Geometry: final body of the model. Coordinates: model frame, mm. Face numbers are marked on the shaded views. A direction names the side the tool comes from. Round coordinates to 2 decimals unless told otherwise and drop trailing zeros. Loops run counter-clockwise (first coordinate to the right, second up) from the corner with the lowest first, then second, coordinate; pieces in that order, holes last. Notation, with made-up numbers: M 3.25,67 L 54.25,67 A25 ccw 54.25,97 Z; hole C 52,-35.5 d3. An arc over 180 degrees is marked long. Answer as a JSON object with one key per item and string values.
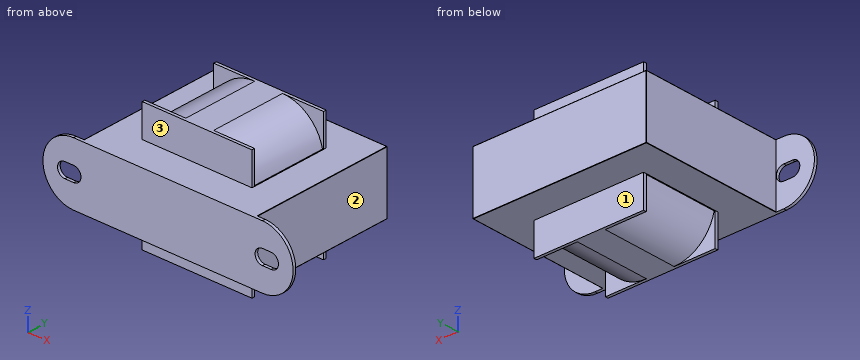
from build123d import *

# Parameters (mm, degrees)
SKETCH1_W           = 59.3
SKETCH1_H           = 48.97
BASE_EXTRUDE_DEPTH  = 10.5
BOSS_EXTRUDE1_DEPTH = 1
CUT_EXTRUDE1_DEPTH  = 10
BOSS_EXTRUDE2_DEPTH = 13
CUT_EXTRUDE2_DEPTH  = 13
SKETCH6_W           = 37.5
SKETCH6_H           = 43
BOSS_EXTRUDE3_DEPTH = 1
SKETCH7_W           = 37.5
SKETCH7_H           = 43
BOSS_EXTRUDE4_DEPTH = 1
FILLET1_R           = 0.1


with BuildPart() as part:
    # Sketch1 → Base-Extrude (new body, symmetric)
    with BuildSketch(Plane.XY):
        with Locations((32.25, 25.485)):
            Rectangle(SKETCH1_W, SKETCH1_H)
    extrude(amount=BASE_EXTRUDE_DEPTH, both=True)

    # Sketch2 → Boss-Extrude1 (add)
    with BuildSketch(Plane.XZ.offset(-1)):
        with BuildLine():
            Line((0, 10.5), (64.5, 10.5))
            ThreePointArc((64.5, 10.5), (75, 0), (64.5, -10.5))
            Line((64.5, -10.5), (0, -10.5))
            ThreePointArc((0, -10.5), (-10.5, 0), (0, 10.5))
        make_face()
    extrude(amount=BOSS_EXTRUDE1_DEPTH)

    # Sketch3 → Cut-Extrude1 (cut)
    with BuildSketch(Plane.XZ):
        with BuildLine():
            Line((64.5, 2.5), (67.5, 2.5))
            ThreePointArc((67.5, 2.5), (70, 0), (67.5, -2.5))
            Line((67.5, -2.5), (64.5, -2.5))
            ThreePointArc((64.5, -2.5), (62, 0), (64.5, 2.5))
        make_face()
        with BuildLine():
            Line((-3, 2.5), (0, 2.5))
            ThreePointArc((0, 2.5), (2.5, 0), (0, -2.5))
            Line((0, -2.5), (-3, -2.5))
            ThreePointArc((-3, -2.5), (-5.5, 0), (-3, 2.5))
        make_face()
    extrude(amount=-CUT_EXTRUDE1_DEPTH, mode=Mode.SUBTRACT)

    # Sketch4 → Boss-Extrude2 (add, symmetric)
    with BuildSketch(Plane(origin=(0, 24.97, 0), x_dir=(-1, 0, 0), z_dir=(0, 1, 0))):
        with BuildLine():
            Line((-37, 21.5), (-27.5, 21.5))
            ThreePointArc((-27.5, 21.5), (-17.600505063, 17.399494937), (-13.5, 7.5))
            Line((-13.5, 7.5), (-13.5, -7.5))
            ThreePointArc((-13.5, -7.5), (-17.600505063, -17.399494937), (-27.5, -21.5))
            Line((-27.5, -21.5), (-37, -21.5))
            ThreePointArc((-37, -21.5), (-46.899494937, -17.399494937), (-51, -7.5))
            Line((-51, -7.5), (-51, 7.5))
            ThreePointArc((-51, 7.5), (-46.899494937, 17.399494937), (-37, 21.5))
        make_face()
    extrude(amount=BOSS_EXTRUDE2_DEPTH, both=True)

    # Sketch5 → Cut-Extrude2 (cut, symmetric)
    with BuildSketch(Plane(origin=(0, 24.97, 0), x_dir=(-1, 0, 0), z_dir=(0, 1, 0))):
        with BuildLine():
            Line((-13.5, 10.5), (-13.825205669, 10.5))
            ThreePointArc((-13.825205669, 10.5), (-13.581538867, 9.008787487), (-13.5, 7.5))
            Line((-13.5, 7.5), (-13.5, 10.5))
        make_face()
        with BuildLine():
            Line((-51, 10.5), (-50.674794331, 10.5))
            ThreePointArc((-50.674794331, 10.5), (-50.918461133, 9.008787487), (-51, 7.5))
            Line((-51, 7.5), (-51, 10.5))
        make_face()
        with BuildLine():
            Line((-51, -10.5), (-50.674794331, -10.5))
            ThreePointArc((-50.674794331, -10.5), (-50.918461133, -9.008787487), (-51, -7.5))
            Line((-51, -7.5), (-51, -10.5))
        make_face()
        with BuildLine():
            Line((-13.5, -10.5), (-13.825205669, -10.5))
            ThreePointArc((-13.825205669, -10.5), (-13.581538867, -9.008787487), (-13.5, -7.5))
            Line((-13.5, -7.5), (-13.5, -10.5))
        make_face()
    extrude(amount=CUT_EXTRUDE2_DEPTH, both=True, mode=Mode.SUBTRACT)

    # Sketch6 → Boss-Extrude3 (add)
    with BuildSketch(Plane(origin=(0, 37.97, 0), x_dir=(-1, 0, 0), z_dir=(0, 1, 0))):
        with Locations((-32.25, 0)):
            Rectangle(SKETCH6_W, SKETCH6_H)
    extrude(amount=BOSS_EXTRUDE3_DEPTH)

    # Sketch7 → Boss-Extrude4 (add)
    with BuildSketch(Plane.XZ.offset(-11.97)):
        with Locations((32.25, 0)):
            Rectangle(SKETCH7_W, SKETCH7_H)
    extrude(amount=BOSS_EXTRUDE4_DEPTH)

    # Fillet1
    fillet1_edges = [part.edges().sort_by_distance(p)[0] for p in [
        (61.9, 25.485, 10.5),
        (32.25, 49.97, 10.5),
        (2.6, 25.485, 10.5),
        (32.25, 49.97, -10.5),
        (61.9, 25.485, -10.5),
        (2.6, 25.485, -10.5),
        (2.6, 49.97, 0),
        (61.9, 49.97, 0),
    ]]
    fillet(fillet1_edges, radius=FILLET1_R)


solid = part.part
1) Section query A-A (z = 0). Return the cut outline in (x, y).
Results:
{"outline": "M -10.5,0 L -5.5,0 L -5.5,1 L -10.5,1 Z; M 2.5,0 L 62,0 L 62,1 L 61.9,1 L 61.9,49.87 A0.1 ccw 61.8,49.97 L 2.7,49.97 A0.1 ccw 2.6,49.87 L 2.6,1 L 2.5,1 Z; M 70,0 L 75,0 L 75,1 L 70,1 Z"}
2) Section query C-C (x = 34). Return the cut outline in (y, z), and give its area (3 significant figures).
Results:
{"outline": "M 0,-10.5 L 10.97,-10.5 L 10.97,-21.5 L 38.97,-21.5 L 38.97,-10.5 L 49.87,-10.5 A0.1 ccw 49.97,-10.4 L 49.97,10.4 A0.1 ccw 49.87,10.5 L 38.97,10.5 L 38.97,21.5 L 10.97,21.5 L 10.97,10.5 L 0,10.5 Z", "area": "1,670 mm2"}
3) Ray query, line 1 (Z direction, x = 23, y = 39); line 2 (X direction, y = 12, z = -0.5); line 3 (Y direction, x = 67, z = -6.5). Return the intervals inside material, ascending.
Results:
{"line 1": "-10.5 to 10.5", "line 2": "2.6 to 61.9", "line 3": "0 to 1"}
4) Section query B-B (y = 14.5). Return the cut outline in (x, z), and give its area (3 significant figures).
Results:
{"outline": "M 2.6,-10.4 A0.1 ccw 2.7,-10.5 L 13.5,-10.5 L 13.5,-7.5 A14 ccw 27.5,-21.5 L 37,-21.5 A14 ccw 51,-7.5 L 51,-10.5 L 61.8,-10.5 A0.1 ccw 61.9,-10.4 L 61.9,10.4 A0.1 ccw 61.8,10.5 L 51,10.5 L 51,7.5 A14 ccw 37,21.5 L 27.5,21.5 A14 ccw 13.5,7.5 L 13.5,10.5 L 2.7,10.5 A0.1 ccw 2.6,10.4 Z", "area": "1,900 mm2"}
5) Pin query (flat end, axial travel): P1, Ø3.5, axis at y = 29.5, z = -9, coming from the +X side; P2, Ø5.5, axis at x = 34, z = -18.5, coming from the -Y side; P3, Ø2.5, axis at y = 18.5, z = 8.5, coming from the -X side. Return the tip coordinate at first contact, or that it passes through.
Results:
{"P1": "x = 61.9", "P2": "y = 10.97", "P3": "x = 2.6"}
6) Reachability of the marked faces 1, 2 and 3 from +Z, -Z, +X, -X, +Y, -Y: full face, straight path, thin tool, end or side. Return the list, or none.
Results:
{"face 1": "-Z, +X, -X, +Y", "face 2": "+Z, -Z, +X, +Y", "face 3": "+Z, +X, -X, -Y"}
7) Section query D-D (z = 17). Return the cut outline in (x, y), and give its area (3 significant figures).
Results:
{"outline": "M 13.5,10.97 L 51,10.97 L 51,11.97 L 47.28,11.97 L 47.28,37.97 L 51,37.97 L 51,38.97 L 13.5,38.97 L 13.5,37.97 L 17.22,37.97 L 17.22,11.97 L 13.5,11.97 Z", "area": "857 mm2"}
